Check sheet for the modelled part. Datum: model origin and axes. Units: mm. Round coordinates to 2 decimals unless told otherwise and drop trailing zeros. Loops run counter-clockwise (first coordinate to the right, second up) from the corner with the lowest first, then second, coordinate; pieces in that order, holes last. Notation, with made-up numbers: M 84,-28.75 L 135,-28.75 A26 cw 135,-9.75 Z; hole C 89,53.5 d9. An arc over 180 degrees is marked long. One line per question, with ' | ' between items. Start each with the question number.
(1) Go/stop test with flat-tipped pins: P1, Ø3, axis at x = 87.5, z = 0, coming from the -Y side; P2, Ø5.5, axis at x = 12.5, z = 0, coming from the +Y side. Record where each tip stops, or that it passes through.
(2) Section check B-B (y = -1.75). Count the separate pieces of the cut face and the enclosed holes in it, and give its area (3 significant figures).
(3) Section check A-A (x = 196.5). Record the boundary of the cut face in (y, z).
(4) Thickness scan on probe 1 along Y at (x, z) = (410.5, 5). Record the ranges inside material, lowest first. Write a range as [from, to].
```python
from build123d import *

# Parameters (mm, degrees)
SKETCH1_W           = 12
SKETCH1_H           = 8
BOSS_EXTRUDE1_DEPTH = 700
CUT_EXTRUDE3_REACH  = 702
SKETCH4_W           = 1.75
SKETCH4_H           = 0.5
SKETCH5_R           = 1.75
CUT_EXTRUDE4_DEPTH  = 9
SKETCH5_3_R         = 3
SKETCH5_3_R_2       = 1.75
CUT_EXTRUDE5_DEPTH  = 4.5
LPATTERN1_COUNT     = 14
LPATTERN1_PITCH     = 25
LPATTERN1_COL_COUNT = 15
LPATTERN1_COL_PITCH = 25
CHAMFER1_SIZE       = 0.25


with BuildPart() as part:
    # Sketch1 → Boss-Extrude1 (new body)
    with BuildSketch(Plane(origin=(0, 0, 0), x_dir=(0, 0, -1), z_dir=(1, 0, 0))):
        Rectangle(SKETCH1_W, SKETCH1_H)
    extrude(amount=BOSS_EXTRUDE1_DEPTH)

    # Sketch4 → Cut-Extrude3 (cut, up to next)
    with BuildSketch(Plane.ZY, mode=Mode.PRIVATE) as cut_extrude3_sk1:
        with Locations((-5.125, 1.75)):
            Rectangle(SKETCH4_W, SKETCH4_H)
    cut_extrude3_tool1 = extrude(cut_extrude3_sk1.sketch, amount=-CUT_EXTRUDE3_REACH, mode=Mode.PRIVATE) & part.part
    add(cut_extrude3_tool1.solids().sort_by_distance((0, 1.75, -5.125))[0], mode=Mode.SUBTRACT)
    # Sketch4 → Cut-Extrude3 (cut, up to next)
    with BuildSketch(Plane.ZY, mode=Mode.PRIVATE) as cut_extrude3_sk2:
        with Locations((5.125, 1.75)):
            Rectangle(SKETCH4_W, SKETCH4_H)
    cut_extrude3_tool2 = extrude(cut_extrude3_sk2.sketch, amount=-CUT_EXTRUDE3_REACH, mode=Mode.PRIVATE) & part.part
    add(cut_extrude3_tool2.solids().sort_by_distance((0, 1.75, 5.125))[0], mode=Mode.SUBTRACT)

    # Sketch5 → Cut-Extrude4 (cut, through all)
    with BuildSketch(Plane(origin=(0, 4, 0), x_dir=(1, 0, 0), z_dir=(0, 1, 0))):
        with Locations((337.5, 0)):
            Circle(SKETCH5_R)
    cut_extrude4 = extrude(amount=-CUT_EXTRUDE4_DEPTH, mode=Mode.SUBTRACT)

    # Sketch5_3 → Cut-Extrude5 (cut)
    with BuildSketch(Plane(origin=(0, 4, 0), x_dir=(1, 0, 0), z_dir=(0, 1, 0))):
        with Locations((337.5, 0)):
            Circle(SKETCH5_3_R)
        with Locations((337.5, 0)):
            Circle(SKETCH5_3_R_2, mode=Mode.SUBTRACT)
    cut_extrude5 = extrude(amount=-CUT_EXTRUDE5_DEPTH, mode=Mode.SUBTRACT)

    # LPattern1: Cut-Extrude4, Cut-Extrude5 ×14
    with Locations(*[(-i * LPATTERN1_PITCH, 0, 0) for i in range(1, LPATTERN1_COUNT)]):
        add(cut_extrude4, mode=Mode.SUBTRACT)
        add(cut_extrude5, mode=Mode.SUBTRACT)

    # LPattern1 col: Cut-Extrude4, Cut-Extrude5 ×15
    with Locations(*[(i * LPATTERN1_COL_PITCH, 0, 0) for i in range(1, LPATTERN1_COL_COUNT)]):
        add(cut_extrude4, mode=Mode.SUBTRACT)
        add(cut_extrude5, mode=Mode.SUBTRACT)

    # Chamfer1
    chamfer1_edges = [part.edges().sort_by_distance(p)[0] for p in [
        (700, -1.25, -6),
        (660.75, -4, 0),
        (685.75, -4, 0),
        (310.75, -4, 0),
        (285.75, -4, 0),
        (260.75, -4, 0),
        (235.75, -4, 0),
        (210.75, -4, 0),
        (700, 4, 0),
        (185.75, -4, 0),
        (160.75, -4, 0),
        (0, 3, -6),
        (135.75, -4, 0),
        (110.75, -4, 0),
        (85.75, -4, 0),
        (60.75, -4, 0),
        (35.75, -4, 0),
        (700, 3, -6),
        (10.75, -4, 0),
        (359.5, 4, 0),
        (384.5, 4, 0),
        (409.5, 4, 0),
        (434.5, 4, 0),
        (350, 1.5, -6),
        (350, 2, -6),
        (459.5, 4, 0),
        (0, 1.5, -5.125),
        (484.5, 4, 0),
        (0, 1.75, -4.25),
        (0, 2, -5.125),
        (509.5, 4, 0),
        (534.5, 4, 0),
        (559.5, 4, 0),
        (584.5, 4, 0),
        (609.5, 4, 0),
        (634.5, 4, 0),
        (659.5, 4, 0),
        (684.5, 4, 0),
        (309.5, 4, 0),
        (284.5, 4, 0),
        (259.5, 4, 0),
        (234.5, 4, 0),
        (0, -1.25, 6),
        (209.5, 4, 0),
        (184.5, 4, 0),
        (159.5, 4, 0),
        (700, -1.25, 6),
        (134.5, 4, 0),
        (109.5, 4, 0),
        (84.5, 4, 0),
        (59.5, 4, 0),
        (34.5, 4, 0),
        (350, 1.5, 6),
        (9.5, 4, 0),
        (350, 2, 6),
        (0, 1.5, 5.125),
        (0, 2, 5.125),
        (0, 1.75, 4.25),
        (700, 3, 6),
        (335.75, -4, 0),
        (0, 4, 0),
        (334.5, 4, 0),
        (0, -1.25, -6),
        (0, -4, 0),
        (360.75, -4, 0),
        (0, 3, 6),
        (385.75, -4, 0),
        (410.75, -4, 0),
        (435.75, -4, 0),
        (700, -4, 0),
        (460.75, -4, 0),
        (350, 4, 6),
        (350, 4, -6),
        (485.75, -4, 0),
        (350, -4, -6),
        (350, -4, 6),
        (510.75, -4, 0),
        (535.75, -4, 0),
        (560.75, -4, 0),
        (585.75, -4, 0),
        (610.75, -4, 0),
        (635.75, -4, 0),
    ]]
    chamfer(chamfer1_edges, length=CHAMFER1_SIZE)


solid = part.part
```
The answers:
1) P1: through | P2: y = -0.5
2) separate pieces: 1 | enclosed holes: 28 | area: 8,130 mm²
3) outline: M -4,-5.75 L -3.75,-6 L 1.25,-6 L 1.5,-5.75 L 1.5,-4.25 L 2,-4.25 L 2,-5.75 L 2.25,-6 L 3.75,-6 L 4,-5.75 L 4,5.75 L 3.75,6 L 2.25,6 L 2,5.75 L 2,4.25 L 1.5,4.25 L 1.5,5.75 L 1.25,6 L -3.75,6 L -4,5.75 Z
4) probe 1: [-4, 1.5], [2, 4]
